Geometry: see drawing. Coordinates: mm, zero at the bounding-box minimum. A direction names the side the tool comes from. Round coordinates to 2 decimals unless told otherwise and drop trailing zeros. Loops run counter-clockwise (first coordinate to the right, second up) from the corner with the lowest first, then second, coordinate; pieces in that order, holes last.
(1) Draft query along Y for the marked faces 4, 5, 6 and 7. Return one class per face: released by +Y, released by -Y, zero draft, split by the parting line, or undercut.
(2) Cut plane D-D, the plane x = 23. Output: boundary loops of the cut face in (y, z) (3 decimals), and give its area (3 significant figures).
(3) Line query: line 1 (Y direction, x = 43, z = 6.25); line 2 (Y direction, x = 43, z = 12.8); line 3 (Z direction, x = 59, y = 14) (3 decimals). Output: solid intervals per line, ascending.
(4) First-contact query: pin 1 Ø5 at (y, z) = (35.5, 10.5) entering from -X; pin 2 Ø8 at (x, y) = (49, 31.5) entering from -Z; pin 3 Ø14.5 at (x, y) = (43, 27) entering from +Z; pin 4 Ø4 at (y, z) = (21.5, 12) entering from +X. Flat tips, straight axial feed; report the tip coordinate or a pass-through.
(5) Access query for the marked faces 1, 2 and 3. Directions: +Z, -Z, +X, -X, +Y, -Y. A direction counts if a zero-diameter tool reaches every point of the face in a straight line with its end or side. Return the directions, or none.
(6) Cut plane C-C, the plane z = 2.75. Output: boundary loops of the cut face in (x, y), and give its area (3 significant figures).
(7) Cut plane A-A, the plane y = 27. Output: boundary loops of the cut face in (x, z) (3 decimals), and give its area (3 significant figures).
(8) Cut plane B-B, the plane x = 43. Output: boundary loops of the cut face in (y, z) (3 decimals).
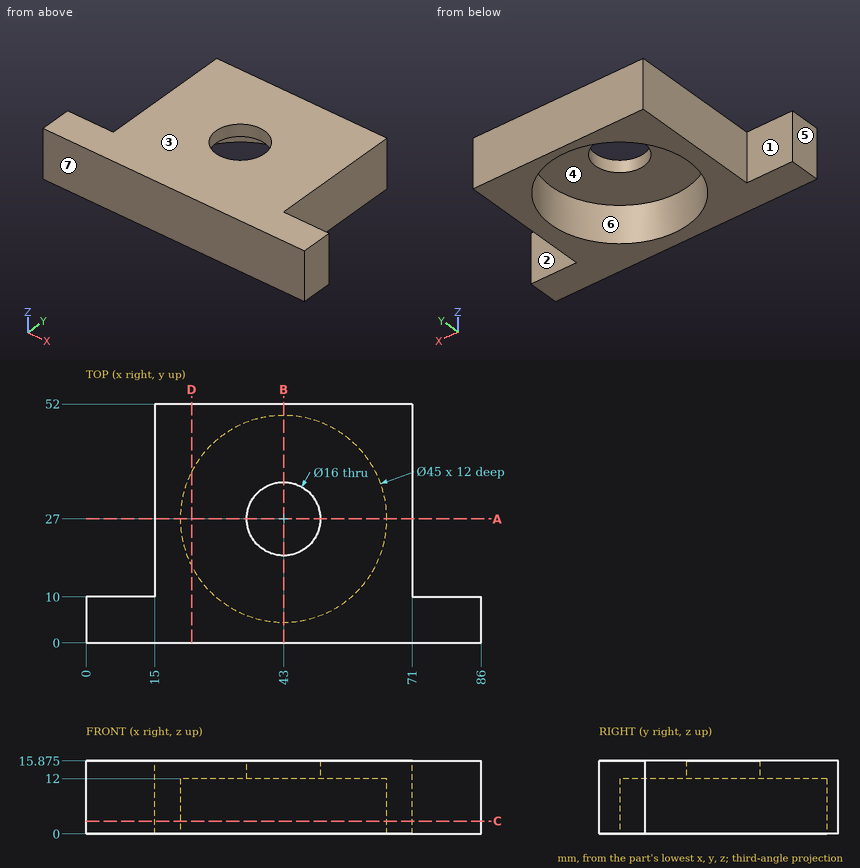
Reported:
1. face 4: undercut
1. face 5: zero draft
1. face 6: undercut
1. face 7: released by -Y
2. outline: (0, 0) - (16.692, 0) - (16.692, 12) - (37.308, 12) - (37.308, 0) - (52, 0) - (52, 15.875) - (0, 15.875) - close
2. area: 578 mm2
3. line 1: y = 0 to 4.5, 49.5 to 52
3. line 2: y = 0 to 19, 35 to 52
3. line 3: z = 12 to 15.875
4. pin 1: stops at x = 15
4. pin 2: stops at z = 12
4. pin 3: passes through
4. pin 4: stops at x = 71
5. face 1: +Z, -Z, -X, +Y
5. face 2: +Z, -Z, +X, +Y
5. face 3: +Z, +X, -X, +Y, -Y
6. outline: (0, 0) - (86, 0) - (86, 10) - (71, 10) - (71, 52) - (15, 52) - (15, 10) - (0, 10) - close; hole circle Ø45 at (43, 27)
6. area: 1,620 mm2
7. outline: (15, 0) - (20.5, 0) - (20.5, 12) - (35, 12) - (35, 15.875) - (15, 15.875) - close; (51, 12) - (65.5, 12) - (65.5, 0) - (71, 0) - (71, 15.875) - (51, 15.875) - close
7. area: 287 mm2
8. outline: (0, 0) - (4.5, 0) - (4.5, 12) - (19, 12) - (19, 15.875) - (0, 15.875) - close; (35, 12) - (49.5, 12) - (49.5, 0) - (52, 0) - (52, 15.875) - (35, 15.875) - close
